from build123d import *

# Parameters (mm, degrees)
SKETCH_1_W          = 22.94
SKETCH_1_H          = 12
EXTRUDE_1_DEPTH     = 4
CUT_EXTRUDE_1_DEPTH = 3
CUT_EXTRUDE_START   = -3
CUT_EXTRUDE_2_DEPTH = 3
CUT_EXTRUDE_4_DEPTH = 2
SKETCH_6_R          = 2
CUT_EXTRUDE_5_DEPTH = 14.548464858
CHAMFER_1_SIZE      = 1
CHAMFER_2_SIZE      = 1
CUT_EXTRUDE_START_2 = 10
SKETCH_7_R          = 2
SKETCH_7_R_2        = 1.8
CUT_EXTRUDE_6_DEPTH = 10
SKETCH_8_R          = 2
SKETCH_8_R_2        = 1.8
CUT_EXTRUDE_7_DEPTH = 3
SKETCH_9_R          = 2.2
CUT_EXTRUDE_8_DEPTH = 14.548464858
CUT_EXTRUDE_9_DEPTH = 2


with BuildPart() as part:
    # Эскиз1 → Бобышка-Вытянуть1 (new body)
    with BuildSketch(Plane.XY):
        Rectangle(SKETCH_1_W, SKETCH_1_H)
    extrude(amount=EXTRUDE_1_DEPTH)

    # Эскиз3 → Вырез-Вытянуть1 (cut)
    with BuildSketch(Plane(origin=(11.47, 0, 0), x_dir=(0, 0, -1), z_dir=(1, 0, 0))):
        with BuildLine():
            ThreePointArc((-4, 0), (-2, 2), (0, 0))
            Line((0, 0), (0, 6))
            Line((0, 6), (-4, 6))
            Line((-4, 6), (-4, 0))
        make_face()
        with BuildLine():
            Line((-4, -6), (0, -6))
            Line((0, -6), (0, 0))
            ThreePointArc((0, 0), (-2, -2), (-4, 0))
            Line((-4, 0), (-4, -6))
        make_face()
    extrude(amount=-CUT_EXTRUDE_1_DEPTH, mode=Mode.SUBTRACT)

    # Эскиз4 → Вырез-Вытянуть2 (cut)
    with BuildSketch(Plane.ZY.offset(11.47).offset(CUT_EXTRUDE_START)):
        with BuildLine():
            Line((4, 6), (0, 6))
            Line((0, 6), (0, 0))
            ThreePointArc((0, 0), (2, 2), (4, 0))
            Line((4, 0), (4, 6))
        make_face()
        with BuildLine():
            ThreePointArc((4, 0), (2, -2), (0, 0))
            Line((0, 0), (0, -6))
            Line((0, -6), (4, -6))
            Line((4, -6), (4, 0))
        make_face()
    extrude(amount=CUT_EXTRUDE_2_DEPTH, mode=Mode.SUBTRACT)

    # Эскиз5 → Вырез-Вытянуть4 (cut)
    with BuildSketch(Plane(origin=(0, 0, 0), x_dir=(-1, 0, 0), z_dir=(0, 0, -1))):
        Polygon((0, -4.041451884), (3.5, -2.020725942), (3.5, 2.020725942), (0, 4.041451884), (-3.5, 2.020725942), (-3.5, -2.020725942), align=None)
    extrude(amount=-CUT_EXTRUDE_4_DEPTH, mode=Mode.SUBTRACT)

    # Эскиз6 → Вырез-Вытянуть5 (cut, through all)
    with BuildSketch(Plane(origin=(0, 0, 0), x_dir=(-1, 0, 0), z_dir=(0, 0, -1))):
        Circle(SKETCH_6_R)
    extrude(amount=-CUT_EXTRUDE_5_DEPTH, mode=Mode.SUBTRACT)

    # Фаска1
    chamfer_1_edges = [part.edges().sort_by_distance(p)[0] for p in [
        (0, 6, 0),
    ]]
    chamfer(chamfer_1_edges, length=CHAMFER_1_SIZE)

    # Фаска2
    chamfer_2_edges = [part.edges().sort_by_distance(p)[0] for p in [
        (0, 6, 4),
        (0, -6, 4),
        (0, -6, 0),
    ]]
    chamfer(chamfer_2_edges, length=CHAMFER_2_SIZE)

    # Эскиз7 → Вырез-Вытянуть6 (cut)
    with BuildSketch(Plane(origin=(8.47, 0, 0), x_dir=(0, 0, -1), z_dir=(1, 0, 0)).offset(CUT_EXTRUDE_START_2)):
        with Locations(Location((-2, 0, 0), (0, 0, 270))):
            Circle(SKETCH_7_R)
        with Locations(Location((-2, 0, 0), (0, 0, 270))):
            Circle(SKETCH_7_R_2, mode=Mode.SUBTRACT)
    extrude(amount=-CUT_EXTRUDE_6_DEPTH, mode=Mode.SUBTRACT)

    # Эскиз8 → Вырез-Вытянуть7 (cut)
    with BuildSketch(Plane.ZY.offset(11.47).offset(CUT_EXTRUDE_START)):
        with Locations((2, 0)):
            Circle(SKETCH_8_R)
        with Locations(Location((2, 0, 0), (0, 0, 270))):
            Circle(SKETCH_8_R_2, mode=Mode.SUBTRACT)
    extrude(amount=CUT_EXTRUDE_7_DEPTH, mode=Mode.SUBTRACT)

    # Эскиз9 → Вырез-Вытянуть8 (cut, through all)
    with BuildSketch(Plane(origin=(0, 0, 0), x_dir=(-1, 0, 0), z_dir=(0, 0, -1))):
        Circle(SKETCH_9_R)
    extrude(amount=-CUT_EXTRUDE_8_DEPTH, mode=Mode.SUBTRACT)

    # Эскиз10 → Вырез-Вытянуть9 (cut)
    with BuildSketch(Plane(origin=(0, 0, 0), x_dir=(-1, 0, 0), z_dir=(0, 0, -1))):
        Polygon((0, -4.272391992), (3.7, -2.136195996), (3.7, 2.136195996), (0, 4.272391992), (-3.7, 2.136195996), (-3.7, -2.136195996), align=None)
    extrude(amount=-CUT_EXTRUDE_9_DEPTH, mode=Mode.SUBTRACT)


solid = part.part
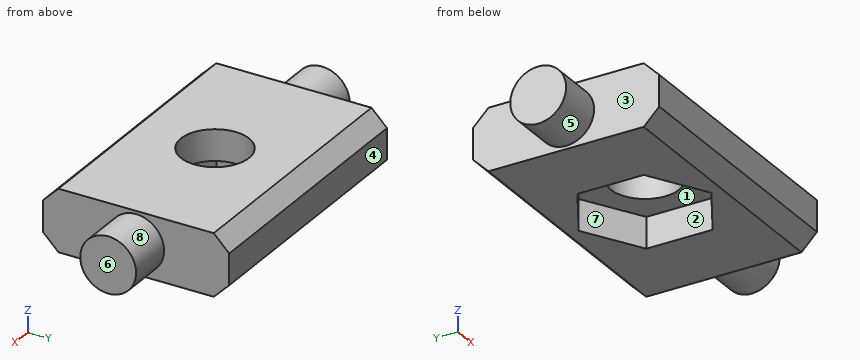
Source: CAD feature listing. Evaluate the final solid. Frame: model axes, mm. Face numbers are marked on the shaded views. A direction names the side the tool comes from. Give positions to 0.01 mm unless a question says otherwise; leave off trailing zeros. Write each loop counter-clockwise with the first axis right and the second up, starting at its lowest first coordinate (ties: lowest second). Pieces come first, ordered by that corner, then holes. Notation, with made-up numbers: M -22.75,33.5 L 12.25,33.5 A13 ccw 12.25,50.5 Z; hole C 58.25,26 d7. An arc over 180 degrees is marked long. Return JSON: item names as keys, results as strings. Group by question number.
1) Cut plane C-C, the plane x = 3. Output: boundary loops of the cut face in (y, z), plus the area to 3 significant figures.
2) Cut plane D-D, the plane y = 3.25. Output: boundary loops of the cut face in (x, z), plus the area to 3 significant figures.
3) Pin query (flat end, axial travel): P1, Ø6, axis at x = 0.5, y = 0, coming from the -Z side. Return the tip coordinate at first contact, or that it passes through.
4) Cut plane A-A, the plane y = 0. Output: boundary loops of the cut face in (x, z), plus the area to 3 significant figures.
5) Cut plane B-B, the plane z = 1.6. Output: boundary loops of the cut face in (x, y) (3 decimals).
6) Set-up query: the marked faces 5, 6, 7 and 8. Return all of +Z, -Z, +X, -X, +Y, -Y with unobstructed straight access to the full face (end or side cutting, diameter ignored); none if empty.
7) Material intervals for line 1 along Y through (x, z) = (0, 2.85); line 2 along X through (y, z) = (5.25, 1.3); line 3 along Y through (x, z) = (-2.5, 1.2), sorted ascending. Write a range as [from, to].
8) Pull-direction query (X, two-part tool) for the marked faces 1, 2, 3 and 4; classes: pulls with the +X half, pulls with the -X half, needs draft (parallel to the pull), parting line crosses it, or undercut.
Recorded:
{
 "1": {"outline": "M -6,1 L -5,0 L -2.54,0 L -2.54,2 L 2.54,2 L 2.54,0 L 5,0 L 6,1 L 6,3 L 5,4 L -5,4 L -6,3 Z", "area": "35.8 mm²"},
 "2": {"outline": "M -8.47,0 L -1.77,0 L -1.77,2 L 1.77,2 L 1.77,0 L 8.47,0 L 8.47,4 L -8.47,4 Z", "area": "60.7 mm²"},
 "3": {"P1": "stops at z = 2"},
 "4": {"outline": "M -11.47,0.2 L -8.47,0.2 L -8.47,0 L -3.7,0 L -3.7,2 L -2.2,2 L -2.2,4 L -8.47,4 L -8.47,3.8 L -11.47,3.8 Z; M 2.2,2 L 3.7,2 L 3.7,0 L 8.47,0 L 8.47,0.2 L 11.47,0.2 L 11.47,3.8 L 8.47,3.8 L 8.47,4 L 2.2,4 Z", "area": "65.8 mm²"},
 "5": {"outline": "M -11.47,-1.755 L -8.47,-1.755 L -8.47,-6 L 8.47,-6 L 8.47,-1.755 L 11.47,-1.755 L 11.47,1.755 L 8.47,1.755 L 8.47,6 L -8.47,6 L -8.47,1.755 L -11.47,1.755 Z; hole M -3.7,-2.136 L 0,-4.272 L 3.7,-2.136 L 3.7,2.136 L 0,4.272 L -3.7,2.136 Z"},
 "6": {"face 5": "-X", "face 6": "+Z, -Z, +X, +Y, -Y", "face 7": "-Z", "face 8": "+X"},
 "7": {"line 1": "y = [-6, -2.2], [2.2, 6]", "line 2": "x = [-8.47, 8.47]", "line 3": "y = [-6, -2.83], [2.83, 6]"},
 "8": {"face 1": "undercut", "face 2": "undercut", "face 3": "pulls with the -X half", "face 4": "needs draft"}
}
